Part print with two shaded views. Sizes in mm from the minimum x, y, z corner. Round coordinates to 2 decimals unless told otherwise and drop trailing zeros. Loops run counter-clockwise (first coordinate to the right, second up) from the corner with the lowest first, then second, coordinate; pieces in that order, holes last. Notation, with made-up numbers: M 15,9.25 L 65,9.25 A22 ccw 65,39.25 Z; hole C 63.5,-39 d2. An arc over 180 degrees is marked long. Answer as CSV lines item,"result". Start each with the question number.
Item 1: Drop a flat-ended pin along its axis: pin 1 Ø2.5 at (x, z) = (89.94, 2.5) entering from -Y. Give the stop position or say it passes through.
Item 2: Band-saw the part on A-A (x = 14). Give the cut face in (y, z), and give its area (3 significant figures).
Item 3: Wall check: line 1 (X direction, y = 0.4, z = 2.5); line 2 (X direction, y = 0.2, z = 33.5); line 3 (Z direction, x = 53, y = 1.4). Give the ranges that are in metal, low to high.
Item 4: Band-saw the part on C-C (x = 56.5). Give the cut face in (y, z).
Item 5: Band-saw the part on D-D (z = 50.5). Give the cut face in (x, y).
Item 6: Band-saw the part on B-B (z = 16.5). Give the cut face in (x, y), and give its area (3 significant figures).
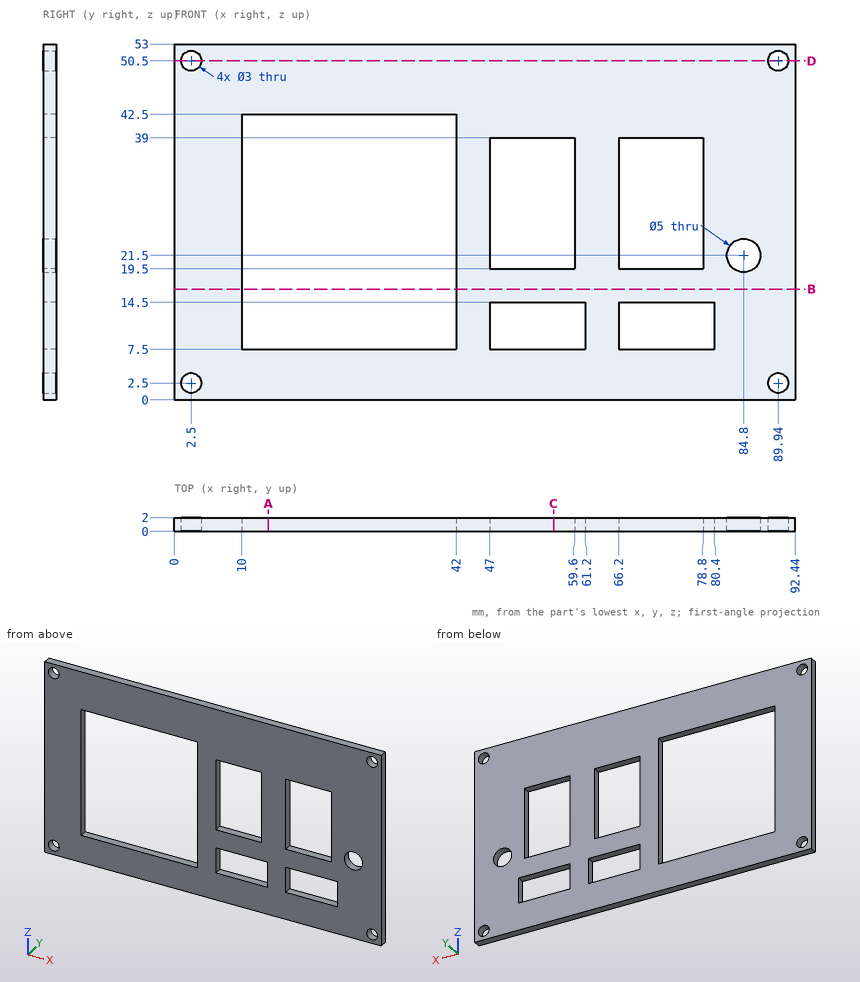
Answer block:
1,pin 1,"passes through"
2,outline,"M 0,0 L 2,0 L 2,7.5 L 0,7.5 Z; M 0,42.5 L 2,42.5 L 2,53 L 0,53 Z"
2,area,"36.0 mm^2"
3,line 1,"x = 0 to 1, 4 to 88.44, 91.44 to 92.44"
3,line 2,"x = 0 to 10, 42 to 47, 59.6 to 66.2, 78.8 to 92.44"
3,line 3,"z = 0 to 7.5, 14.5 to 19.5, 39 to 53"
4,outline,"M 0,0 L 2,0 L 2,7.5 L 0,7.5 Z; M 0,14.5 L 2,14.5 L 2,19.5 L 0,19.5 Z; M 0,39 L 2,39 L 2,53 L 0,53 Z"
5,outline,"M 0,0 L 1,0 L 1,2 L 0,2 Z; M 4,0 L 88.44,0 L 88.44,2 L 4,2 Z; M 91.44,0 L 92.44,0 L 92.44,2 L 91.44,2 Z"
6,outline,"M 0,0 L 10,0 L 10,2 L 0,2 Z; M 42,0 L 92.44,0 L 92.44,2 L 42,2 Z"
6,area,"121 mm^2"
